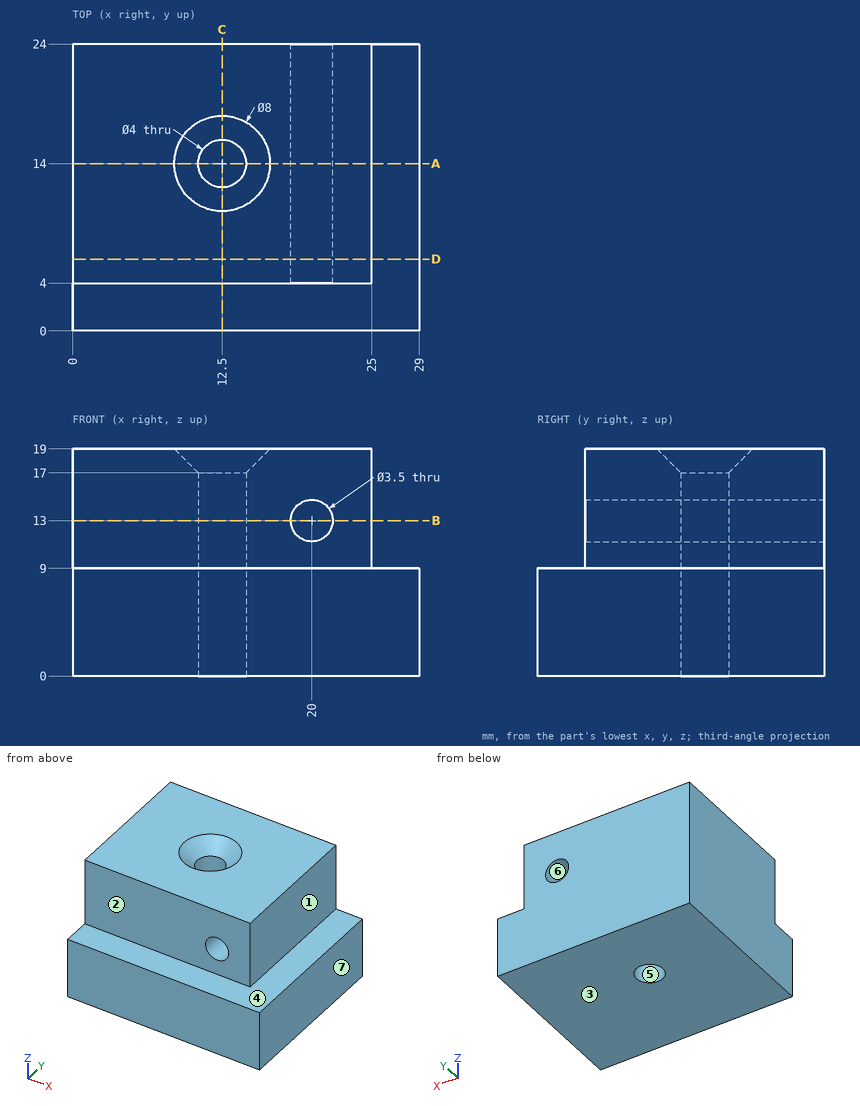
Verification items for this drawing (mm, ordinates from the low corner). A direction names the side the tool comes from. Coordinates: 2 decimals unless noted, no trailing zeros. Order: outer loops, then holes, each group sorted by start corner. A loop starts at its lowest first (then second) coordinate and runs counter-clockwise, first axis right, second up.
Q1. Draft check along X on the marked faces 4, 5, 6 and 7. Enter one of: released by +X, released by -X, zero draft, split by the parting line, or undercut.
Reply:
face 4: zero draft
face 5: undercut
face 6: undercut
face 7: released by +X
Q2. Depth check by flat-ended pin: pin 1 Ø3 at (x, z) = (20, 13) entering from -Y; pin 2 Ø10 at (y, z) = (10, 16) entering from +X. Enter the tip coordinate at first touch or a pass-through.
Reply:
pin 1: passes through
pin 2: stops at x = 25
Q3. Sectioned sample at B-B on z = 13. Record the cut outline in (x, y), and give its area (3 significant figures).
Reply:
outline: (0, 4) - (18.25, 4) - (18.25, 24) - (0, 24) - close; (21.75, 4) - (25, 4) - (25, 24) - (21.75, 24) - close; hole circle Ø4 at (12.5, 14)
area: 417 mm2
Q4. Sectioned sample at C-C on x = 12.5. Record the cut outline in (y, z), and give its area (3 significant figures).
Reply:
outline: (0, 0) - (12, 0) - (12, 17) - (10, 19) - (4, 19) - (4, 9) - (0, 9) - close; (16, 0) - (24, 0) - (24, 19) - (18, 19) - (16, 17) - close
area: 336 mm2
Q5. Sectioned sample at D-D on y = 6. Record the cut outline in (x, z).
Reply:
outline: (0, 0) - (29, 0) - (29, 9) - (25, 9) - (25, 19) - (0, 19) - close; hole circle Ø3.5 at (20, 13)
Q6. Thickness scan on probe 1 along Z at (x, y) = (20, 18.25); probe 2 along X at (y, z) = (14, 8.75); probe 3 along Y at (x, z) = (12.5, 7). Record the ranges inside material, lowest first.
Reply:
probe 1: z = 0 to 11.25, 14.75 to 19
probe 2: x = 0 to 10.5, 14.5 to 29
probe 3: y = 0 to 12, 16 to 24
Q7. Tool access check on the marked faces 1, 2 and 3. Record the directions out of +Z, -Z, +X, -X, +Y, -Y that give a thin tool (end or side, any length) a straight path to the whole face; none if there is none.
Reply:
face 1: +Z, +X, +Y, -Y
face 2: +Z, +X, -X, -Y
face 3: -Z, +X, -X, +Y, -Y
Q8. Sectioned sample at A-A on y = 14. Record the cut outline in (x, z).
Reply:
outline: (0, 0) - (10.5, 0) - (10.5, 17) - (8.5, 19) - (0, 19) - close; (14.5, 0) - (29, 0) - (29, 9) - (25, 9) - (25, 19) - (16.5, 19) - (14.5, 17) - close; hole circle Ø3.5 at (20, 13)
